Autodesk Inventor part; units mm, degrees
ref_plane "YZ Plane" through (0, 0, 0) normal (1, 0, 0) x (0, 1, 0)
ref_plane "XZ Plane" through (0, 0, 0) normal (0, 1, 0) x (-1, 0, 0)
ref_plane "XY Plane" through (0, 0, 0) normal (0, 0, 1) x (1, 0, 0)
sketch "スケッチ1" plane through (0, 0, 0) normal (1, 0, 0) x (0, 1, 0)
  line L0 (3, 22.53) -> (-3, 22.53)
  line L1 (-3, 22.53) -> (-3, -22.53)
  line L2 (-3, -22.53) -> (3, -22.53)
  line L3 (3, -22.53) -> (3, 22.53)
  line L4 (0, 22.53) -> (0, -22.53) construction
  line L5 (3, 0) -> (-3, 0) construction
  arc A0 (0.9953, 1.1222) -> (-0.9953, 1.1222) centre (0, 3.47) ccw
  arc A1 (-0.9953, -1.1222) -> (0.9953, -1.1222) centre (0, -3.47) ccw
  arc A2 (-0.9953, 1.1222) -> (-0.9953, -1.1222) centre (0, 0) ccw
  arc A3 (0.9953, -1.1222) -> (0.9953, 1.1222) centre (0, 0) ccw
  dimension "d0" = 6
  dimension "d1" = 45.06
  dimension "d3" = 5.1
  dimension "d4" = 12.04
  dimension "d5" = 1.5
extrude "押し出し1" add sketch "スケッチ1" along normal mid plane 9.3
sketch "スケッチ2" plane through (-4.65, 3, 22.53) normal (0, 1, 0) x (1, 0, 0)
  line L0 (4.65, 0) -> (4.65, 45.06) construction
  line L1 (9.3, 0) -> (0, 0) construction
  circle A0 centre (4.65, 4.23) radius 1.5
  circle A1 centre (4.65, 11.63) radius 1.5
  line L2 (9.3, 23.6522) -> (9.3, 21.4078) construction
  line L3 (9.3, 22.53) -> (-0.0401, 22.53) construction
  line L4 (9.3, 45.06) -> (0, 45.06) construction
  circle A2 centre (4.65, 40.83) radius 1.5
  circle A3 centre (4.65, 33.43) radius 1.5
  point P0 (4.65, 22.53)
  dimension "d8" = 21.8
  dimension "d9" = 7.4
  dimension "d10" = 3
extrude "押し出し2" cut sketch "スケッチ2" against normal blind 6
chamfer "面取り1" distance 0.75 angle 45 8 edges at (-1.5, 3, 18.3) (-1.5, 3, 10.9) (-1.5, 3, -10.9) (-1.5, 3, -18.3) (-1.5, -3, 18.3) (-1.5, -3, 10.9) (-1.5, -3, -10.9) (-1.5, -3, -18.3)
sketch "スケッチ4" plane through (4.65, 3, -22.53) normal (0, 0, -1) x (-1, 0, 0)
  line L0 (4.65, -3) -> (4.65, -4) construction
  circle A0 centre (4.65, -4) radius 1
  line L1 (9.3, 0) -> (0, 0) construction
  dimension "d19" = 2
  dimension "d20" = 1
  dimension "d21" = 3
extrude "押し出し4" cut sketch "スケッチ4" against normal blind 11.5
properties part number "20_020_LOAD_CELL_R2" material "アルミニウム 6061"
Build history of the part. All positions in model axes, mm. A direction names the side the tool comes from. Round coordinates to 2 decimals unless told otherwise and drop trailing zeros. Loops run counter-clockwise (first coordinate to the right, second up) from the corner with the lowest first, then second, coordinate; pieces in that order, holes last. Notation, with made-up numbers: M 68.5,-5.5 L 107.5,-5.5 A25 ccw 107.5,7.5 Z; hole C 63,-27 d8. An arc over 180 degrees is marked long. Answer as CSV lines item,"result".
1. Cut at D-D on x = 0. Count the separate pieces of the cut face and the enclosed holes in it, then the cut area to 3 significant figures.
Resolved:
separate pieces,"7"
enclosed holes,"1"
area,"133 mm²"
2. Two-plate mould, pull along Y, no slides. Class faces 1 (the cylindrical face through (-0.1, -1.5, 0)), 2 (the cylindrical face through (0.806, 0.031, 17.035)), 3 (the flat face through (0, -3, 0)): released by +Y, released by -Y, zero draft, split by the parting line, or undercut.
Resolved:
face 1,"undercut"
face 2,"zero draft"
face 3,"released by -Y"
3. Cut at C-C on x = -4. Write the cut outline in (y, z), then the cut area to 3 significant figures.
Resolved:
outline,"M -3,-22.53 L 3,-22.53 L 3,22.53 L -3,22.53 Z; hole M -1,-1.12 A2.55 ccw long 1,-1.12 A1.5 ccw 1,1.12 A2.55 ccw long -1,1.12 A1.5 ccw Z"
area,"224 mm²"
4. Cut at A-A on z = 0. Write the cut outline in (x, y), then the cut area to 3 significant figures.
Resolved:
outline,"M -4.65,-3 L 4.65,-3 L 4.65,-1.5 L -4.65,-1.5 Z; M -4.65,1.5 L 4.65,1.5 L 4.65,3 L -4.65,3 Z"
area,"27.9 mm²"
5. Wall check: probe 1 along Y at (x, z) = (0.25, 3.47); probe 2 along X at (y, z) = (-1, -21.8); probe 3 along Z at (x, y) = (-1, 0.6). Give the ranges that are in metal, low to high. Write a range as [from, to].
Resolved:
probe 1,"y = [-3, -2.55], [2.55, 3]"
probe 2,"x = [-4.65, -1], [1, 4.65]"
probe 3,"z = [-22.53, -19.42], [-17.18, -12.02], [-9.78, -5.95], [5.95, 9.78], [12.02, 17.18], [19.42, 22.53]"
6. Cut at B-B on y = -0.6. Write the cut outline in (x, z).
Resolved:
outline,"M -4.65,-22.53 L -0.92,-22.53 L -0.92,-19.49 A1.5 cw -0.92,-17.11 L -0.92,-12.09 A1.5 cw long 0.92,-12.09 L 0.92,-17.11 A1.5 cw 0.92,-19.49 L 0.92,-22.53 L 4.65,-22.53 L 4.65,-5.95 L -4.65,-5.95 Z; M -4.65,5.95 L 4.65,5.95 L 4.65,22.53 L -4.65,22.53 Z; hole C 0,10.9 d3; hole C 0,18.3 d3"
7. Flat gauge pin, fed straight in: P1, Ø1.2, axis at x = 0, y = -1, coming from the -Z side. Where does the tip first touch, or does it go through?
Resolved:
P1,"stops at z = -9.53"
8. 3-axis set-ups, long thin cutter, end or side, ignore diameter. For faces 4 (the cylindrical face through (-0.07, -0.1, 6.02)), 5 (the cylindrical face through (1, -1, -15)): which of +Z, -Z, +X, -X, +Y, -Y reach the whole face in a straight line?
Resolved:
face 4,"+X, -X"
face 5,"-Z"
